from build123d import *

# Parameters (mm, degrees)
SKETCH1_R           = 13.6525
SKETCH1_R_2         = 10.668
BOSS_EXTRUDE1_DEPTH = 25.4
BOSS_EXTRUDE2_REACH = 55.786
SKETCH4_R           = 12.7
SKETCH4_R_2         = 10.668
SKETCH12_R          = 10.668
CUT_EXTRUDE1_DEPTH  = 19.05
BOSS_EXTRUDE4_REACH = 41.064


with BuildPart() as part:
    # Sketch1 → Boss-Extrude1 (new body)
    with BuildSketch(Plane(origin=(0, 0, 0), x_dir=(1, 0, 0), z_dir=(0, 1, 0))):
        with Locations(Location((0, 0, 0), (0, 0, 270))):
            Circle(SKETCH1_R)
        with Locations(Location((0, 0, 0), (0, 0, 270))):
            Circle(SKETCH1_R_2, mode=Mode.SUBTRACT)
    extrude(amount=BOSS_EXTRUDE1_DEPTH)

    # Sketch10 → Cut-Revolve4 (revolve, cut)
    with BuildSketch(Plane(origin=(0, 0, 0), x_dir=(0, 0, -1), z_dir=(1, 0, 0)), mode=Mode.PRIVATE) as cut_revolve4_sk:
        Polygon((-13.6525, 0), (-13.6525, 3.81), (-12.7, 0), align=None)
    cut_revolve4 = revolve(cut_revolve4_sk.sketch.rotate(Axis((0, 0, 0), (0, 1, 0)), 180), axis=Axis((0, 0, 0), (0, 1, 0)), mode=Mode.SUBTRACT)

    # Mirror1: Cut-Revolve4 across plane
    add(cut_revolve4.mirror(Plane.ZX.offset(12.7)), mode=Mode.SUBTRACT)

    # Sketch4 → Boss-Extrude2 (add, up to next)
    with BuildSketch(Plane.XY.offset(-31.75), mode=Mode.PRIVATE) as boss_extrude2_sk1:
        with Locations(Location((0, 12.7, 0), (0, 0, 224.427003928))):
            Circle(SKETCH4_R)
        with Locations(Location((0, 12.7, 0), (0, 0, 236.442690207))):
            Circle(SKETCH4_R_2, mode=Mode.SUBTRACT)
    boss_extrude2_tool1 = extrude(boss_extrude2_sk1.sketch, amount=BOSS_EXTRUDE2_REACH, mode=Mode.PRIVATE) - part.part
    add(boss_extrude2_tool1.solids().sort_by_distance((8.813087, 21.338553, -31.75))[0])

    # Sketch11 → Cut-Revolve5 (revolve, cut)
    with BuildSketch(Plane(origin=(0, 0, 0), x_dir=(0, 0, -1), z_dir=(1, 0, 0)), mode=Mode.PRIVATE) as cut_revolve5_sk:
        Polygon((31.75, 0), (27.94, 0), (31.75, 0.9525), align=None)
    revolve(cut_revolve5_sk.sketch.rotate(Axis((0, 12.7, -31.75), (0, 0, 1)), 270), axis=Axis((0, 12.7, -31.75), (0, 0, 1)), mode=Mode.SUBTRACT)

    # Sketch12 → Cut-Extrude1 (cut)
    with BuildSketch(Plane(origin=(0, 0, -31.75), x_dir=(-1, 0, 0), z_dir=(0, 0, -1))):
        with Locations(Location((0, 12.7, 0), (0, 0, 303.557309793))):
            Circle(SKETCH12_R)
    extrude(amount=-CUT_EXTRUDE1_DEPTH, mode=Mode.SUBTRACT)

    # Sketch13 → Boss-Extrude4 (add, up to next)
    with BuildSketch(Plane(origin=(0, 0, -12.7), x_dir=(-1, 0, 0), z_dir=(0, 0, -1)), mode=Mode.PRIVATE) as boss_extrude4_sk1:
        with BuildLine():
            ThreePointArc((4.42238726, 2.991822265), (10.668, 12.700000001), (4.422387259, 22.408177735))
            add(Edge.make_bspline(
                [(4.422387248, 22.408177726), (4.714008579, 22.02457668), (5.010065494, 21.59)],
                knots=[0.341540519, 0.341540519, 0.341540519, 0.384917679, 0.384917679, 0.384917679], degree=2, weights=[1, 1.000235206, 1]))
            Line((5.010065494, 21.59), (5.010065494, 20.65120417))
            ThreePointArc((5.010065494, 20.65120417), (9.398, 12.7), (5.010065494, 4.74879583))
            Line((5.010065494, 4.74879583), (5.010065494, 3.81))
            add(Edge.make_bspline(
                [(5.010065496, 3.810000003), (4.714008581, 3.375423322), (4.422387248, 2.991822274)],
                knots=[-0.384917679, -0.384917679, -0.384917679, -0.341540519, -0.341540519, -0.341540519], degree=2, weights=[1, 1.000235206, 1]))
        make_face()
    boss_extrude4_tool1 = extrude(boss_extrude4_sk1.sketch, amount=-BOSS_EXTRUDE4_REACH, mode=Mode.PRIVATE) - part.part
    # Sketch13 → Boss-Extrude4 (add, up to next)
    with BuildSketch(Plane(origin=(0, 0, -12.7), x_dir=(-1, 0, 0), z_dir=(0, 0, -1)), mode=Mode.PRIVATE) as boss_extrude4_sk2:
        with BuildLine():
            add(Edge.make_bspline(
                [(-5.010065494, 21.59), (-4.714008579, 22.02457668), (-4.422387248, 22.408177726)],
                knots=[-0.384917679, -0.384917679, -0.384917679, -0.341540519, -0.341540519, -0.341540519], degree=2, weights=[1, 1.000235206, 1]))
            ThreePointArc((-4.422387259, 22.408177735), (-10.668, 12.7), (-4.422387258, 2.991822265))
            add(Edge.make_bspline(
                [(-4.422387248, 2.991822273), (-4.71400858, 3.375423321), (-5.010065496, 3.810000003)],
                knots=[0.341540519, 0.341540519, 0.341540519, 0.384917679, 0.384917679, 0.384917679], degree=2, weights=[1, 1.000235206, 1]))
            Line((-5.010065494, 3.81), (-5.010065494, 4.74879583))
            ThreePointArc((-5.010065494, 4.74879583), (-9.398, 12.7), (-5.010065494, 20.65120417))
            Line((-5.010065494, 20.65120417), (-5.010065494, 21.59))
        make_face()
    boss_extrude4_tool2 = extrude(boss_extrude4_sk2.sketch, amount=-BOSS_EXTRUDE4_REACH, mode=Mode.PRIVATE) - part.part
    add(boss_extrude4_tool1.solids().sort_by_distance((-10.464039, 12.7, -12.7))[0])
    add(boss_extrude4_tool2.solids().sort_by_distance((5.214027, 21.120602, -12.7))[0])


solid = part.part
Here's how the part is built. I have some questions about the finished solid (model axes, mm). A direction names the side the tool comes from. Coordinates: 2 decimals unless noted, no trailing zeros. Write each loop counter-clockwise with the first axis right and the second up, starting at its lowest first coordinate (ties: lowest second). Pieces come first, ordered by that corner, then holes.
1) I'm going to push flat-ended pins straight in: pin 1 (10 mm diameter, centred on x = 0.5, y = 15, fed in from -Z); pin 2 (1.5 mm diameter, centred on y = 9, z = -19, fed in from +X); pin 3 (12 mm diameter, centred on y = 21.5, z = 7.5, fed in from -X). Where does each tip first touch, or does it pass through?
Filled in:
pin 1: stops at z = -12.7
pin 2: stops at x = 12.35
pin 3: stops at x = -13.57
2) Thinking about a two-plate mould opening in Z: for faces 3 (the face through (-6.491, 12.522, -8.466)), 4 (the face through (-10.4, 15.9, -31.75)), 5 (the face through (-6.712, 23.481, -19.183)), which applies, +Z half, -Z half, draft (parallel to the pull), parting line (faces both ways), or undercut?
Filled in:
face 3: undercut
face 4: -Z half
face 5: draft
3) If we section it at A-A (z = 0): List the corners of the cut face in (x, y) for me, plus the area to 3 significant figures.
Filled in:
outline: (-13.65, 3.81) - (-12.7, 0) - (-10.67, 0) - (-10.67, 25.4) - (-12.7, 25.4) - (-13.65, 21.59) - close; (10.67, 0) - (12.7, 0) - (13.65, 3.81) - (13.65, 21.59) - (12.7, 25.4) - (10.67, 25.4) - close
area: 144 mm2
4) If I drill on line 1 (X direction, y = 11.5, z = 0); line 2 (Y direction, x = 0, z = -23); line 3 (X direction, y = 12.7, z = -21.5), over which ranges is the centre line in solid material (lowest first)?
Filled in:
line 1: x = -13.65 to -10.67, 10.67 to 13.65
line 2: y = 0 to 2.03, 23.37 to 25.4
line 3: x = -12.7 to -10.67, 10.67 to 12.7
5) Which directions (+Z, -Z, +X, -X, +Y, -Y) give clear straight access to the entire face, cutting with the end or side of a thin tool? Please do faces 1 (the face through (-0.56, 25.215, 12.734)), 2 (the face through (0, 13, -12.7)).
Filled in:
face 1: +Y
face 2: -Z
6) If we section it at C-C (z = -24): List the corners of the cut face in (x, y) for me, plus the area to 3 significant figures.
Filled in:
outline: circle Ø25.4 at (0, 12.7); hole circle Ø21.34 at (0, 12.7)
area: 149 mm2
